Read the model definition and answer for the solid it produces. Units are mm, in the model's axes. A direction names the side the tool comes from. Round coordinates to 2 decimals unless told otherwise and drop trailing zeros. Write each loop counter-clockwise with the first axis right and the second up, starting at its lowest first coordinate (ties: lowest second). Pieces come first, ordered by that corner, then holes. Notation, with made-up numbers: (-32.75, 36) - (-8.75, 36) arc R13 cw to (-8.75, 45) - close; hole circle Ø10 at (1.25, -11.75). An arc over 180 degrees is marked (long way). One line per item, written item: value. Start each with the question number.
(1) The mould has two halves that part along Z. Classify faces 3 (the face through (-103, 2, -33)), 4 (the face through (-102.88, 0.99, 23.92)), 5 (the face through (-1, 0, 0)): +Z half, -Z half, draft (parallel to the pull), parting line (faces both ways), or undercut.
(2) A cutting plane is placed at A-A, the plane y = 1.35. Determine the outline of the cut face in (x, z), plus the area to 3 significant figures.
(3) Flat-ended cylindrical pins translate along their axes: pin 1 Ø8.5 at (x, z) = (94.5, 30) entering from +Y; pin 2 Ø5 at (x, z) = (95, 28) entering from -Y. Find the tip coordinate at first contact, or state that the pin passes through.
(4) Find the intervals of material crossed by L1, parallel to X at y = 2.7, z = -25; L2, parallel to X at y = 1.45, z = 25; L3, parallel to X at y = 1.2, z = 29, in increasing order.
(5) For faces 1 (the face through (102, 2, 34)), 2 (the face through (93.5, 2, -29)), determine the directions among +Z, -Z, +X, -X, +Y, -Y from which every point of the face is accessible in a straight line to the end or side of a thin tool.
from build123d import *

# Parameters (mm, degrees)
SKETCH1_W           = 208
SKETCH1_H           = 70
SKETCH1_R           = 1.25
BOSS_EXTRUDE1_DEPTH = 3
FILLET1_R           = 5
SKETCH2_R           = 5
SKETCH2_R_2         = 4.75
CUT_EXTRUDE2_DEPTH  = 2


with BuildPart() as part:
    # Sketch1 → Boss-Extrude1 (new body)
    with BuildSketch(Plane(origin=(0, 0, 0), x_dir=(1, 0, 0), z_dir=(0, 1, 0))):
        Rectangle(SKETCH1_W, SKETCH1_H)
        with Locations(Location((-98, 25, 0), (0, 0, 270))):
            Circle(SKETCH1_R, mode=Mode.SUBTRACT)
        with Locations(Location((-98, -25, 0), (0, 0, 270))):
            Circle(SKETCH1_R, mode=Mode.SUBTRACT)
        with Locations(Location((94.5, 30, 0), (0, 0, 270))):
            Circle(SKETCH1_R, mode=Mode.SUBTRACT)
        with Locations(Location((94.5, -30, 0), (0, 0, 270))):
            Circle(SKETCH1_R, mode=Mode.SUBTRACT)
    extrude(amount=BOSS_EXTRUDE1_DEPTH)

    # Fillet1
    fillet1_edges = [part.edges().sort_by_distance(p)[0] for p in [
        (104, 1.5, 35),
        (-104, 1.5, 35),
        (-104, 1.5, -35),
        (104, 1.5, -35),
    ]]
    fillet(fillet1_edges, radius=FILLET1_R)

    # Sketch2 → Cut-Extrude2 (cut)
    with BuildSketch(Plane(origin=(0, 0, 0), x_dir=(1, 0, 0), z_dir=(0, 1, 0))):
        with Locations(Location((-98, 25, 0), (0, 0, 270))):
            Circle(SKETCH2_R)
        with Locations(Location((94.5, 30, 0), (0, 0, 270))):
            Circle(SKETCH2_R_2)
        with Locations(Location((94.5, -30, 0), (0, 0, 270))):
            Circle(SKETCH2_R_2)
        with Locations(Location((-98, -25, 0), (0, 0, 270))):
            Circle(SKETCH2_R)
    extrude(amount=CUT_EXTRUDE2_DEPTH, mode=Mode.SUBTRACT)


solid = part.part
Here are the results:
1. face 3: -Z half
1. face 4: undercut
1. face 5: draft
2. outline: (-104, -30) arc R5 ccw to (-99, -35) - (99, -35) arc R5 ccw to (104, -30) - (104, 30) arc R5 ccw to (99, 35) - (-99, 35) arc R5 ccw to (-104, 30) - close; hole circle Ø10 at (-98, -25); hole circle Ø10 at (-98, 25); hole circle Ø9.5 at (94.5, -30); hole circle Ø9.5 at (94.5, 30)
2. area: 14,200 mm²
3. pin 1: y = 3
3. pin 2: y = 2
4. L1: -104 to -99.25, -96.75 to 104
4. L2: -104 to -103, -93 to 104
4. L3: -104 to -101, -95 to 89.86, 99.14 to 104
5. face 1: +Z, +X, +Y, -Y
5. face 2: -Y
